from build123d import *

# Parameters (mm, degrees)
F1_DEPTH = 8
F2_R     = 1.5
F3_DEPTH = 25
F4_R     = 2.75
F5_DEPTH = 3
F6_R     = 5


with BuildPart() as f1:
    # F0 (on Front) → F1 (new body)
    with BuildSketch(Plane.XZ):
        with BuildLine():
            Line((-33, -24.75), (-33, -79.052559))
            Line((-33, -79.052559), (33, -79.052559))
            Line((33, -79.052559), (33, -24.75))
            ThreePointArc((33, -24.75), (39.133186, -13.044395), (41.25, 0))
            ThreePointArc((41.25, 0), (36.25, 5), (31.25, 0))
            ThreePointArc((31.25, 0), (0, -31.25), (-31.25, 0))
            ThreePointArc((-31.25, 0), (-36.25, 5), (-41.25, 0))
            ThreePointArc((-41.25, 0), (-39.133186, -13.044395), (-33, -24.75))
        make_face()
    extrude(amount=F1_DEPTH)

    # F2 (on face) → F3 (cut)
    with BuildSketch(Plane.XZ.offset(8)):
        with Locations((18, -42.60355)):
            Circle(F2_R)
        with Locations((-18, -42.60355)):
            Circle(F2_R)
        with Locations((-18, -67.60355)):
            Circle(F2_R)
        with Locations((18, -67.60355)):
            Circle(F2_R)
    extrude(amount=-F3_DEPTH, mode=Mode.SUBTRACT)

    # F4 (on face) → F5 (cut)
    with BuildSketch(Plane.XZ.offset(8)):
        with Locations((-18, -42.60355)):
            Circle(F4_R)
        with Locations((18, -42.60355)):
            Circle(F4_R)
        with Locations((18, -67.60355)):
            Circle(F4_R)
        with Locations((-18, -67.60355)):
            Circle(F4_R)
    extrude(amount=-F5_DEPTH, mode=Mode.SUBTRACT)

    # F6
    f6_edges = [f1.edges().sort_by_distance(p)[0] for p in [
        (33, -4, -79.052559),
        (-33, -4, -79.052559),
    ]]
    fillet(f6_edges, radius=F6_R)


solid = f1.part
Verification items for the finished model (mm, model axes). A direction names the side the tool comes from. Give positions to 0.01 mm unless a question says otherwise; leave off trailing zeros. Loops run counter-clockwise (first coordinate to the right, second up) from the corner with the lowest first, then second, coordinate; pieces in that order, holes last.
1) Draft check along X on faces 1 (the cylindrical face through (-31.574, -4.056, -77.549)), 2 (the cylindrical face through (-18.596, -6.521, -70.288)), 3 (the cylindrical face through (31.496, -4.056, -77.627)), 4 (the flat face through (-17, -5, -44)). Enter one of: pulls with the +X half, pulls with the -X half, needs draft (parallel to the pull), parting line crosses it, or undercut.
2) Sectioned sample at C-C, the plane y = -2.75. Enter the section's corners in (x, z).
3) Thickness scan on line 1 along Z through (x, y) = (-18, -1.85); line 2 along Z through (x, y) = (-18, -6.65); line 3 along X through (y, z) = (-6.25, -68.5). Record the ranges inside material, lowest first.
4) Sectioned sample at A-A, the plane z = -4.5. Enter the section's corners in (x, y).
5) Sectioned sample at B-B, the plane x = 18. Enter the section's corners in (y, z).
6) Sectioned sample at D-D, the plane x = -25. Enter the section's corners in (y, z), then the cut area to 3 significant figures.
7) Depth check by flat-ended pin: pin 1 Ø4 at (y, z) = (-2, -33) entering from -X; pin 2 Ø2.5 at (y, z) = (-3, -51.5) entering from +X; pin 3 Ø1 at (y, z) = (-1.5, -20) entering from +X; pin 4 Ø2 at (x, z) = (-20.5, -19.5) entering from -Y. Enter the tip coordinate at first touch or a pass-through.
8) Set-up check for faces 5 (the flat face through (19, -5, -44)), 6 (the cylindrical face through (-36.14, -3.94, 5)): record each of +Z, -Z, +X, -X, +Y, -Y from which the full face is reachable in a straight line by a thin tool's end or side.
Answers:
1. face 1: pulls with the -X half
1. face 2: undercut
1. face 3: pulls with the +X half
1. face 4: undercut
2. outline: (-41.25, 0) arc R41.25 ccw to (-33, -24.75) - (-33, -74.05) arc R5 ccw to (-28, -79.05) - (28, -79.05) arc R5 ccw to (33, -74.05) - (33, -24.75) arc R41.25 ccw to (41.25, 0) arc R5 ccw to (31.25, 0) arc R31.25 cw to (-31.25, 0) arc R5 ccw to start; hole circle Ø3 at (-18, -67.6); hole circle Ø3 at (-18, -42.6); hole circle Ø3 at (18, -67.6); hole circle Ø3 at (18, -42.6)
3. line 1: z = -79.05 to -69.1, -66.1 to -44.1, -41.1 to -25.55
3. line 2: z = -79.05 to -70.35, -64.85 to -45.35, -39.85 to -25.55
3. line 3: x = -33 to -20.6, -15.4 to 15.4, 20.6 to 33
4. outline: (-41, -8) - (-30.92, -8) - (-30.92, 0) - (-41, 0) - close; (30.92, -8) - (41, -8) - (41, 0) - (30.92, 0) - close
5. outline: (-8, -79.05) - (0, -79.05) - (0, -69.1) - (-5, -69.1) - (-5, -70.35) - (-8, -70.35) - close; (-8, -64.85) - (-5, -64.85) - (-5, -66.1) - (0, -66.1) - (0, -44.1) - (-5, -44.1) - (-5, -45.35) - (-8, -45.35) - close; (-8, -39.85) - (-5, -39.85) - (-5, -41.1) - (0, -41.1) - (0, -25.55) - (-8, -25.55) - close
6. outline: (-8, -79.05) - (0, -79.05) - (0, -18.75) - (-8, -18.75) - close
6. area: 482 mm2
7. pin 1: stops at x = -33
7. pin 2: stops at x = 33
7. pin 3: stops at x = 36.35
7. pin 4: passes through
8. face 5: -Y
8. face 6: +Z, +Y, -Y
